Read the model definition and answer for the solid it produces. Units are mm, in the model's axes. A direction names the side the tool comes from. Round coordinates to 2 decimals unless told otherwise and drop trailing zeros. Loops run counter-clockwise (first coordinate to the right, second up) from the corner with the lowest first, then second, coordinate; pieces in that order, holes last. Notation, with made-up numbers: M 77.5,78 L 83.5,78 A22 cw 83.5,111 Z; hole C 75.5,64.5 d4. An arc over 180 degrees is marked long. Write each question's results on one line, items separated by ' | '.
```python
from build123d import *

# Parameters (mm, degrees)
BOSS_EXTRUDE2_START   = -76.2
SKETCH3_W             = 15.875
SKETCH3_H             = 25.4
BOSS_EXTRUDE2_DEPTH   = 6.35
SKETCH4_W             = 38.1
SKETCH4_H             = 7.874
SKETCH4_R             = 1.016
BOSS_EXTRUDE3_DEPTH   = 3.175
BOSS_EXTRUDE3_2_DEPTH = 3.175
BOSS_EXTRUDE4_REACH   = 85.527
BOSS_EXTRUDE5_DEPTH   = 25.4
BOSS_EXTRUDE7_DEPTH   = 25.4
BOSS_EXTRUDE8_START   = -19.05
BOSS_EXTRUDE8_DEPTH   = 7.874
BOSS_EXTRUDE8_START_2 = 11.176
BOSS_EXTRUDE8_2_DEPTH = 7.874
SKETCH9_R             = 1.89865
CUT_EXTRUDE2_DEPTH    = 3.81
SKETCH10_R            = 3.175
CUT_EXTRUDE3_DEPTH    = 96.846325291


with BuildPart() as part:
    # Sketch3 → Boss-Extrude2 (new body)
    with BuildSketch(Plane(origin=(0, 0, 0), x_dir=(0, 0, -1), z_dir=(1, 0, 0)).offset(BOSS_EXTRUDE2_START)):
        with Locations((0, 25.4)):
            Rectangle(SKETCH3_W, SKETCH3_H)
    extrude(amount=BOSS_EXTRUDE2_DEPTH)



with BuildPart() as body_2:
    # Sketch4 → Boss-Extrude3 (new body)
    with BuildSketch(Plane(origin=(0, 0, 0), x_dir=(-0.7071067811865477, 0.7071067811865475, 0), z_dir=(-0.7071067811865475, -0.7071067811865477, 0))):
        with Locations((0, -15.113)):
            Rectangle(SKETCH4_W, SKETCH4_H)
        with Locations((13.97, -13.97)):
            Circle(SKETCH4_R, mode=Mode.SUBTRACT)
        with Locations((-13.97, -13.97)):
            Circle(SKETCH4_R, mode=Mode.SUBTRACT)
    extrude(amount=BOSS_EXTRUDE3_DEPTH)

    # Boss-Extrude4: up to this face of the body (flat: up to its plane)
    boss_extrude4_end = Plane(body_2.part.faces().sort_by_distance((0, 0, 15.13825721))[0])
    # Sketch6 → Boss-Extrude4 (add, up to the picked face)
    with BuildSketch(Plane.XZ.offset(-12.7), mode=Mode.PRIVATE) as boss_extrude4_sk1:
        Polygon((-13.470384182, -19.05), (-15.715448212, -19.05), (-15.715448212, -11.176), (-13.470384182, -11.176), (13.470384182, -11.176), (13.470384182, -19.05), align=None)
    boss_extrude4_tool1 = split(extrude(boss_extrude4_sk1.sketch, amount=BOSS_EXTRUDE4_REACH, mode=Mode.PRIVATE), bisect_by=boss_extrude4_end, keep=Keep.BOTH, mode=Mode.PRIVATE)
    # Sketch6 → Boss-Extrude4 (add, up to the picked face)
    with BuildSketch(Plane.XZ.offset(-12.7), mode=Mode.PRIVATE) as boss_extrude4_sk2:
        Polygon((-13.470384182, 11.176), (-15.715448212, 11.176), (-15.715448212, 19.05), (-13.470384182, 19.05), (13.470384182, 19.05), (13.470384182, 11.176), align=None)
    boss_extrude4_tool2 = split(extrude(boss_extrude4_sk2.sketch, amount=BOSS_EXTRUDE4_REACH, mode=Mode.PRIVATE), bisect_by=boss_extrude4_end, keep=Keep.BOTH, mode=Mode.PRIVATE)


with BuildPart() as body_3:
    # Sketch4 → Boss-Extrude3 2 (new body)
    with BuildSketch(Plane(origin=(0, 0, 0), x_dir=(-0.7071067811865477, 0.7071067811865475, 0), z_dir=(-0.7071067811865475, -0.7071067811865477, 0))):
        with Locations((0, 15.113)):
            Rectangle(SKETCH4_W, SKETCH4_H)
        with Locations((13.97, 13.97)):
            Circle(SKETCH4_R, mode=Mode.SUBTRACT)
        with Locations((-13.97, 13.97)):
            Circle(SKETCH4_R, mode=Mode.SUBTRACT)
    extrude(amount=BOSS_EXTRUDE3_2_DEPTH)


with BuildPart() as body_2_1:
    add(body_2.part)

    add(body_3.part)  # Boss-Extrude4 merges body 3
    add(boss_extrude4_tool1.solids().sort_by(Axis((-1.122532, 12.7, -15.113), (0, -1, 0)))[0])
    add(boss_extrude4_tool2.solids().sort_by(Axis((-1.122532, 12.7, 15.113), (0, -1, 0)))[0])

    # Sketch6<2> → Boss-Extrude5 (add)
    with BuildSketch(Plane.XZ.offset(-12.7)):
        Polygon((-13.470384182, -19.05), (-15.715448212, -19.05), (-15.715448212, -11.176), (-13.470384182, -11.176), (13.470384182, -11.176), (13.470384182, -19.05), align=None)
        Polygon((-13.470384182, 11.176), (-15.715448212, 11.176), (-15.715448212, 19.05), (-13.470384182, 19.05), (13.470384182, 19.05), (13.470384182, 11.176), align=None)
    extrude(amount=-BOSS_EXTRUDE5_DEPTH)


with BuildPart() as part_1:
    add(part.part)

    add(body_2_1.part)  # Boss-Extrude7 merges body 2
    # Sketch7 → Boss-Extrude7 (add)
    with BuildSketch(Plane(origin=(0, 38.1, 0), x_dir=(1, 0, 0), z_dir=(0, 1, 0))):
        Polygon((-15.715448212, 19.05), (-76.2, 7.9375), (-76.2, -7.9375), (-15.715448212, -19.05), (-15.715448212, -11.176), (-69.85, 0), (-15.715448212, 11.176), align=None)
    extrude(amount=-BOSS_EXTRUDE7_DEPTH)

    # Boss-Extrude8: read off the stored shape, not the designer's step
    # Boss-Extrude8 outline → Boss-Extrude8 (add)
    with BuildSketch(Plane.XY.offset(BOSS_EXTRUDE8_START)):
        Polygon((-14.240768363, 12.7), (-17.190128061, 12.7), (-15.715448212, 11.225320151), align=None)
    extrude(amount=BOSS_EXTRUDE8_DEPTH)

    # Boss-Extrude8 2 outline → Boss-Extrude8 2 (add)
    with BuildSketch(Plane.XY.offset(BOSS_EXTRUDE8_START_2)):
        Polygon((-14.240768363, 12.7), (-17.190128061, 12.7), (-15.715448212, 11.225320151), align=None)
    extrude(amount=BOSS_EXTRUDE8_2_DEPTH)

    # Sketch9 → Cut-Extrude2 (cut)
    with BuildSketch(Plane.ZY.offset(76.2)):
        with Locations((0, 25.4)):
            Circle(SKETCH9_R)
    extrude(amount=-CUT_EXTRUDE2_DEPTH, mode=Mode.SUBTRACT)

    # Sketch10 → Cut-Extrude3 (cut, through all)
    with BuildSketch(Plane.ZY.offset(72.39)):
        with Locations((0, 25.4)):
            Circle(SKETCH10_R)
    extrude(amount=-CUT_EXTRUDE3_DEPTH, mode=Mode.SUBTRACT)


solid = part_1.part
```
1. Given P1, Ø19, axis at x = -43.5, z = -0.5, coming from the -Y side; P2, Ø5, axis at x = -27.5, y = 10.5, coming from the +Z side; P3, Ø6, axis at y = 25.4, z = 0, coming from the +X side, each flat-ended and moving along its own axis, determine where each tip first touches the part or whether it passes through.
Completed:
P1: stops at y = 12.7 | P2: stops at z = 17.1 | P3: stops at x = -72.39
2. Determine the mould class of faces 1 (the face through (-45.534, 25.578, -13.572)), 2 (the face through (-42.404, 25.578, 5.666)), 3 (the face through (-3.18, -1.31, 15.06)), 4 (the face through (8.93, -11.14, 14.96)) for opening direction Z: released by +Z, released by -Z, zero draft, split by the parting line, or undercut.
Completed:
face 1: released by -Z | face 2: undercut | face 3: zero draft | face 4: undercut
3. Find section C-C, the plane x = -24.5. Give the vertices of the cut face in (y, z).
Completed:
outline: M 12.7,-17.44 L 38.1,-17.44 L 38.1,-9.36 L 12.7,-9.36 Z; M 12.7,9.36 L 38.1,9.36 L 38.1,17.44 L 12.7,17.44 Z
4. Which of the six approach directions +Z, -Z, +X, -X, +Y, -Y give full straight-line access (tool end or side, diameter ignored) to faces 5 (the face through (-53, 12.7, 4)), 6 (the face through (1, 18, 19.05)), 7 (the face through (-72.39, 23, 0))?
Completed:
face 5: +Z, -Z, -X, -Y | face 6: +Z, +X, -X, +Y, -Y | face 7: +X
5. Find the intervals of material crossed by L1, parallel to Z at x = -7.5, y = 31; L2, parallel to Y at x = -75, z = 0; L3, parallel to Z at x = -68, y = 30, in increasing order.
Completed:
L1: z = -19.05 to -11.18, 11.18 to 19.05 | L2: y = 12.7 to 23.5, 27.3 to 38.1 | L3: z = -9.44 to -0.38, 0.38 to 9.44
6. Find section B-B, the plane x = -2.5. Give the vertices of the cut face in (y, z), then the cut area to 3 significant figures.
Completed:
outline: M -1.99,-19.05 L 38.1,-19.05 L 38.1,-11.18 L -1.99,-11.18 Z; M -1.99,11.18 L 38.1,11.18 L 38.1,19.05 L -1.99,19.05 Z | area: 631 mm2
7. Find section D-D, the plane z = -16. Give the vertices of the cut face in (x, y), then the cut area to 3 significant figures.
Completed:
outline: M -32.32,12.7 L -17.19,12.7 L 11.23,-15.72 L 13.47,-13.47 L 13.47,38.1 L -32.32,38.1 Z | area: 1,630 mm2
